Autodesk Fusion 360 part; units mm, degrees
sketch "Sketch1" plane through (0, 0, 0) normal (0, 1, 0) x (1, 0, 0)
  line L0 (0, 0) -> (65, 0)
  line L1 (65, 0) -> (65, 5)
  line L2 (65, 5) -> (80, 5)
  line L3 (80, 5) -> (80, -35)
  line L4 (80, -35) -> (0, -35)
  line L5 (0, -35) -> (-15, -35)
  line L6 (-15, -35) -> (-15, 5)
  line L7 (-15, 5) -> (0, 5)
  line L8 (0, 5) -> (0, 0)
  line L9 (32.5, 0) -> (32.5, -35) construction
  line L10 (32.5, 0) -> (4.5, 0) construction
  line L11 (32.5, 0) -> (60.5, 0) construction
  line L12 (60.5, 0) -> (60.5, -17) construction
  line L13 (56.5, -17) -> (8.5, -17)
  line L14 (4.5, -21) -> (4.5, -35)
  line L15 (60.5, -21) -> (60.5, -35)
  arc A0 (8.5, -17) -> (4.5, -21) centre (8.5, -21) ccw
  arc A1 (60.5, -21) -> (56.5, -17) centre (56.5, -21) ccw
  point P0 (4.5, -17)
  dimension "d1" = 65
  dimension "d2" = 28
  dimension "d3" = 28
  dimension "d4" = 17
  dimension "d5" = 56
  dimension "d6" = 4
  dimension "d7" = 4
extrude "Extrude1" add sketch "Sketch1" along normal blind 50 contours L0 L1 L2 L3 L4 L5 L6 L7 L8 L13 L14 L15 A0 A1
sketch "Sketch2" plane through (0, 0, 35) normal (0, 0, 1) x (1, 0, 0)
  line L0 (-15, 0) -> (4.5, 0)
  line L1 (4.5, 0) -> (4.5, 50)
  line L2 (4.5, 50) -> (-15, 50)
  line L3 (-15, 50) -> (-15, 0)
  line L4 (-15, 25) -> (80, 25) construction
  line L5 (32.5, 0.0866) -> (32.5, 50) construction
  line L6 (32.5, 25) -> (72.5, 25) construction
  line L7 (72.5, 25) -> (72.5, 41.75) construction
  line L8 (72.5, 25) -> (72.5, 8.25) construction
  line L9 (72.5, 41.75) -> (-7.5, 41.75) construction
  line L10 (72.5, 8.25) -> (-7.5, 8.25) construction
  point P0 (-7.5, 41.75)
  point P1 (72.5, 41.75)
  point P2 (72.5, 8.25)
  point P3 (-7.5, 8.25)
  dimension "d10" = 40
  dimension "d11" = 16.75
  dimension "d12" = 16.75
  dimension "d13" = 80
  dimension "d14" = 80
hole "Hole1" at (-7.5, 41.75, 35) at (72.5, 41.75, 35) at (72.5, 8.25, 35) at (-7.5, 8.25, 35) direction (0, 0, -1) diameter 5.5 depth 40 tip angle 118 counterbore diameter 9 counterbore depth 22
sketch "Sketch3" plane through (80, 0, 0) normal (1, 0, 0) x (0, 0, -1)
  line L0 (-35, 0) -> (5, 0)
  line L1 (5, 0) -> (5, 50)
  line L2 (5, 50) -> (-35, 50)
  line L3 (-35, 50) -> (-35, 0)
  line L4 (5, 25) -> (-35, 25) construction
  line L5 (-28.6189, 25) -> (-28.6189, 33) construction
  line L6 (-28.6189, 33) -> (-28.6189, 17) construction
  point P0 (-28.6189, 33)
  point P1 (-28.6189, 17)
hole "Hole2" at (80, 17, 28.6189) at (80, 33, 28.6189) direction (-1, 0, 0) diameter 4.9 depth 40 tip angle 118 counterbore diameter 7 counterbore depth 10
For this review, take the finished solid that the model builds, in its own axes (mm). A direction names the side the tool comes from. Round coordinates to 2 decimals unless told otherwise and drop trailing zeros. Write each loop counter-clockwise with the first axis right and the second up, starting at its lowest first coordinate (ties: lowest second). Pieces come first, ordered by that corner, then holes. Notation, with made-up numbers: (-29.75, 52.5) - (-17.75, 52.5) arc R32 ccw to (-17.75, 84.5) - close; hole circle Ø8 at (68.5, 58). An arc over 180 degrees is marked (long way). Write item = value, one per line. Start each with the question number.
1. For pin 1 Ø5 at (x, y) = (-7.5, 8.25) entering from +Z; pin 2 Ø3 at (x, y) = (50.5, 23) entering from -Z; pin 3 Ø2 at (x, y) = (14.5, 17) entering from +Z, all flat-tipped, find the tip position at first contact; note any pin that passes through.
2. Consider section C-C on y = 8.25. Give the number of separate pieces and of enclosed holes in the cut face, plus the area to 3 significant figures.
3. For faces 4 (the face through (70, 19.3, 27.1)), 5 (the face through (-8.852, 3.958, 23.846)), 6 (the face through (65, 25, -2)), 7 (the face through (60.5, 25, 28)), 8 (the face through (69.773, 8.608, 3.874)), list the 3-axis set-ups (+Z, -Z, +X, -X, +Y, -Y) from which the entire face can be reached by the end or side of a thin tool; tool diameter is ignored.
4. Draft analysis for pull direction X (two halves, no side actions). For faces 1 (the face through (4.5, 25, 28)), 2 (the face through (80, 25, 15)), 3 (the face through (32, 0, 15)), state which applies: released by +X, released by -X, zero draft, split by the parting line, or undercut.
5. Consider section A-A on z = -1. State the section outline as (x, y) points.
6. Consider section D-D on z = 7.5. State the section outline as (x, y) points, plus the area to 3 significant figures.
7. Consider section B-B on y = 33. State the section outline as (x, z) points.
8. Wall thickness on L1, parallel to X at y = 41.75, z = 23.75; L2, parallel to X at y = 8.25, z = -0.5; L3, parallel to Y at x = -7.5, z = 23.5: over which ranges is each line inside the solid? List them lowest first.
Evaluation:
q1.pin_1 = through
q1.pin_2 = 0
q1.pin_3 = 17
q2.separate_pieces = 3
q2.enclosed_holes = 0
q2.area = 1,880 mm2
q3.face_4 = +X
q3.face_5 = +Z
q3.face_6 = -Z, +Y, -Y
q3.face_7 = +Z, +Y, -Y
q3.face_8 = +Z, -Z
q4.face_1 = undercut
q4.face_2 = released by +X
q4.face_3 = zero draft
q5.outline = (-15, 0) - (0, 0) - (0, 50) - (-15, 50) - close; (65, 0) - (80, 0) - (80, 50) - (65, 50) - close; hole circle Ø5.5 at (-7.5, 8.25); hole circle Ø5.5 at (-7.5, 41.75); hole circle Ø5.5 at (72.5, 8.25); hole circle Ø5.5 at (72.5, 41.75)
q6.outline = (-15, 0) - (80, 0) - (80, 50) - (-15, 50) - close; hole circle Ø5.5 at (-7.5, 8.25); hole circle Ø5.5 at (-7.5, 41.75); hole circle Ø5.5 at (72.5, 8.25); hole circle Ø5.5 at (72.5, 41.75)
q6.area = 4,650 mm2
q7.outline = (-15, -5) - (0, -5) - (0, 0) - (65, 0) - (65, -5) - (80, -5) - (80, 25.12) - (70, 25.12) - (70, 26.17) - (60.5, 26.17) - (60.5, 21) arc R4 cw to (56.5, 17) - (8.5, 17) arc R4 cw to (4.5, 21) - (4.5, 35) - (-15, 35) - close; (60.5, 31.07) - (70, 31.07) - (70, 32.12) - (80, 32.12) - (80, 35) - (60.5, 35) - close
q8.L1 = -15 to -12, -3 to 4.5, 60.5 to 68, 77 to 80
q8.L2 = -15 to -10.25, -4.75 to 0, 65 to 69.75, 75.25 to 80
q8.L3 = 0 to 3.75, 12.75 to 37.25, 46.25 to 50
